CAD build for the part. Positions are in the model's coordinates, mm. A direction names the side the tool comes from. Coordinates: 2 decimals unless noted, no trailing zeros. Order: outer loops, then holes, each group sorted by start corner. A loop starts at its lowest first (then second) coordinate and runs counter-clockwise, first axis right, second up. Notation, with made-up numbers: (-10, 40) - (46, 40) arc R34 cw to (46, 73) - close; hole circle Ø6 at (0.25, -4). An arc over 180 degrees is marked (long way). Write each question's results on one line, items separated by ' | '. Start each with the question number.
Q1. Band-saw the part on A-A, the plane x = 31.5. Write the cut outline in (y, z) (3 decimals).
Q2. Pin check, flat tip, straight feed: P1, Ø5, axis at x = 31.5, y = 10, coming from the +Z side. Stop position of the tip, or through.
Q3. Wall check: probe 1 along Y at (x, z) = (31.5, 4.6); probe 2 along Y at (x, z) = (10, 3.95) (3 decimals); probe 3 along X at (y, z) = (10.5, 2.7). Give the ranges that are in metal, low to high.
Q4. Band-saw the part on D-D, the plane x = 10. Write the cut outline in (y, z) (3 decimals).
Q5. Which spindle directions (+Z, -Z, +X, -X, +Y, -Y) get a long thin tool onto all of the face, cutting with end or side? Do faces 1 (the flat face through (0, 10, 2)), 2 (the cylindrical face through (27.504, 10.176, 4.507)). Say none if no direction does.
Q6. Band-saw the part on C-C, the plane z = 2.65. Write the cut outline in (x, y) (3 decimals).
Q7. Band-saw the part on B-B, the plane y = 10. Write the cut outline in (x, z) (3 decimals), then the cut area to 3 significant figures.
Autodesk Inventor part; units mm, degrees
ref_plane "YZ Plane" through (0, 0, 0) normal (1, 0, 0) x (0, 1, 0)
ref_plane "XZ Plane" through (0, 0, 0) normal (0, 1, 0) x (-1, 0, 0)
ref_plane "XY Plane" through (0, 0, 0) normal (0, 0, 1) x (1, 0, 0)
sketch "Sketch1" plane through (0, 0, 0) normal (0, 0, 1) x (1, 0, 0)
  line L0 (0, 0) -> (41.5, 0)
  line L1 (41.5, 0) -> (41.5, 20)
  line L2 (41.5, 20) -> (0, 20)
  line L3 (0, 20) -> (0, 0)
  circle A0 centre (31.5, 10) radius 2.175
  circle A1 centre (10, 10) radius 1.675
  line L4 (20, 20) -> (20, 0) construction
  point P0 (41.5, 10)
  dimension "d0" = 41.5
  dimension "d1" = 4.35
  dimension "d2" = 3.35
  dimension "d3" = 20
  dimension "d4" = 10
  dimension "d5" = 10
  dimension "d6" = 11.5
extrude "Extrusion1" add sketch "Sketch1" along normal blind 5
sketch "Sketch2" plane through (0, 0, 5) normal (0, 0, 1) x (1, 0, 0)
  circle A0 centre (31.5, 10) radius 2.175
  circle A1 centre (31.5, 10) radius 4
  point P0 (0, 0)
  dimension "d9" = 8
extrude "Extrusion2" cut sketch "Sketch2" against normal blind 1
fillet "Fillet1" radius 2 4 edges at (0, 20, 2.5) (41.5, 20, 2.5) (41.5, 0, 2.5) (0, 0, 2.5)
properties part number "PSU_bracket"
Results below:
1) outline: (0, 0) - (7.825, 0) - (7.825, 4) - (6, 4) - (6, 5) - (0, 5) - close; (12.175, 0) - (20, 0) - (20, 5) - (14, 5) - (14, 4) - (12.175, 4) - close
2) P1: stops at z = 4
3) probe 1: y = 0 to 6, 14 to 20 | probe 2: y = 0 to 8.325, 11.675 to 20 | probe 3: x = 0 to 8.4, 11.6 to 29.38, 33.62 to 41.5
4) outline: (0, 0) - (8.325, 0) - (8.325, 5) - (0, 5) - close; (11.675, 0) - (20, 0) - (20, 5) - (11.675, 5) - close
5) face 1: +Z, -Z, -X, +Y, -Y | face 2: +Z
6) outline: (0, 2) arc R2 ccw to (2, 0) - (39.5, 0) arc R2 ccw to (41.5, 2) - (41.5, 18) arc R2 ccw to (39.5, 20) - (2, 20) arc R2 ccw to (0, 18) - close; hole circle Ø3.35 at (10, 10); hole circle Ø4.35 at (31.5, 10)
7) outline: (0, 0) - (8.325, 0) - (8.325, 5) - (0, 5) - close; (11.675, 0) - (29.325, 0) - (29.325, 4) - (27.5, 4) - (27.5, 5) - (11.675, 5) - close; (33.675, 0) - (41.5, 0) - (41.5, 5) - (35.5, 5) - (35.5, 4) - (33.675, 4) - close | area: 165 mm²
